from build123d import *

# Parameters (mm, degrees)
CUT_EXTRUDE1_DEPTH = 2


with BuildPart() as part:
    # Sketch1 → Revolve1 (revolve)
    with BuildSketch(Plane(origin=(0, 0, 0), x_dir=(0, 0, -1), z_dir=(1, 0, 0))):
        with BuildLine():
            Line((0, 0), (0, 3.1))
            Line((0, 3.1), (0.4, 3.5))
            Line((0.4, 3.5), (3.765, 3.5))
            Line((3.765, 3.5), (4, 3.265))
            Line((4, 3.265), (4, 2.35))
            ThreePointArc((4, 2.35), (4.035614876, 2.236081032), (4.129775312, 2.162734164))
            Line((4.129775312, 2.162734164), (4.529775312, 2.012734164))
            ThreePointArc((4.529775312, 2.012734164), (4.564315039, 2.00320929), (4.6, 2))
            Line((4.6, 2), (15.65, 2))
            Line((15.65, 2), (16, 1.65))
            Line((16, 1.65), (16, 0))
            Line((16, 0), (0, 0))
        make_face()
    revolve(axis=Axis((0, 0, 0), (0, 0, -1)))

    # Sketch2 → Cut-Extrude1 (cut)
    with BuildSketch(Plane.XY):
        Polygon((0, 1.732050808), (-1.5, 0.866025404), (-1.5, -0.866025404), (0, -1.732050808), (1.5, -0.866025404), (1.5, 0.866025404), align=None)
    extrude(amount=-CUT_EXTRUDE1_DEPTH, mode=Mode.SUBTRACT)

    # Sketch3 → Cut-Revolve2 (revolve, cut)
    with BuildSketch(Plane(origin=(0, 0, 0), x_dir=(0, 0, -1), z_dir=(1, 0, 0))):
        Polygon((2, 0), (2, 1.5), (2.866025404, 0), align=None)
    revolve(axis=Axis((0, 0, -2), (0, 0, -1)), mode=Mode.SUBTRACT)

    # Sketch4 → Cut-Revolve3 (revolve, cut)
    with BuildSketch(Plane(origin=(0, 0, 0), x_dir=(0, 0, -1), z_dir=(1, 0, 0))):
        Polygon((0, 1.732050808), (0, 1.5), (0.062177826, 1.5), align=None)
    revolve(axis=Axis((0, 0, 0), (0, 0, -1)), mode=Mode.SUBTRACT)


solid = part.part
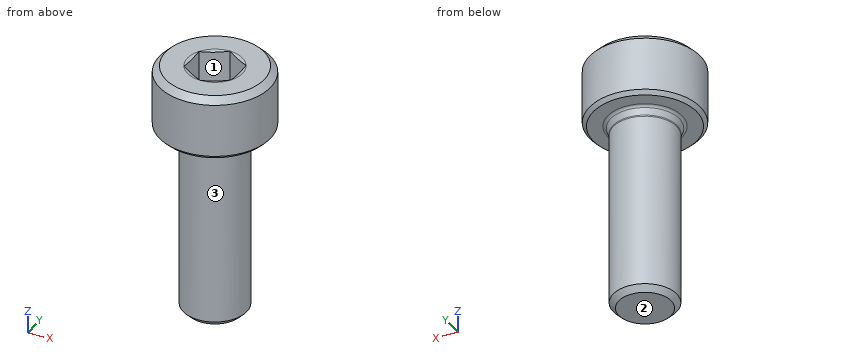
Could you check a few things on this model? Use its own coordinates, in mm. Face numbers are marked on the shaded views. A direction names the side the tool comes from. Round coordinates to 2 decimals unless told otherwise and drop trailing zeros. Order: outer loops, then holes, each group sorted by start corner. A loop starts at its lowest first (then second) coordinate and runs counter-clockwise, first axis right, second up.
(1) Imagine slicing it at A-A (z = -9). Write out the boundary of the cut face in (x, y).
Response values:
outline: circle Ø4 at (0, 0)
(2) Which directions (+Z, -Z, +X, -X, +Y, -Y) give clear straight access to the entire face, cutting with the end or side of a thin tool? Please do the marked faces 1, 2 and 3.
Response values:
face 1: +Z
face 2: -Z, +X, -X, +Y, -Y
face 3: -Z
(3) I'm going to push flat-ended pins straight in: pin 1 (1 mm diameter, centred on y = -2, z = -8, fed in from -X); pin 2 (3 mm diameter, centred on x = 1, z = -13, fed in from -Y); pin 3 (4 mm diameter, centred on x = 2.5, z = -12.5, fed in from +Y). Where does each tip first touch, or does it pass through?
Response values:
pin 1: stops at x = -1.32
pin 2: stops at y = -2
pin 3: stops at y = 1.94
(4) Please list where these lines run through material, in increasing order: line 1 along Y through (x, z) = (1, -9.75); line 2 along Z through (x, y) = (2, 2).
Response values:
line 1: y = -1.73 to 1.73
line 2: z = -4 to 0
